The listing builds one solid part. Answer for the finished solid, in the listing's coordinates (mm). Coordinates: 2 decimals unless noted, no trailing zeros. Order: outer loops, then holes, each group sorted by start corner. A loop starts at its lowest first (then second) coordinate and runs counter-clockwise, first axis right, second up. Notation, with made-up numbers: (-36, 81.25) - (22, 81.25) arc R13 ccw to (22, 103.25) - close; hole circle Ø2 at (48, 0). An arc over 180 degrees is marked (long way). One line per item, written item: value. Start each with the question number.
```python
from build123d import *

# Parameters (mm, degrees)
F0_W     = 152.4
F0_H     = 14.740049
F0_H_2   = 8.316415
F0_H_3   = 8.693536
F1_DEPTH = 3.175
F2_DEPTH = 55.118
F3_W     = 38.1
F3_H     = 9.525
F4_DEPTH = 25.4


with BuildPart() as f1:
    # F0 (on Top) → F1 (new body)
    with BuildSketch(Plane.XY):
        with Locations((77.322651, 15.686439)):
            Rectangle(F0_W, F0_H)
        with Locations((77.322651, 4.158207)):
            Rectangle(F0_W, F0_H_2)
        with Locations((77.322651, -4.346768)):
            Rectangle(F0_W, F0_H_3)
    extrude(amount=F1_DEPTH)

    # F0 (on Top) → F2 (cut)
    with BuildSketch(Plane.XY):
        with Locations((77.322651, 4.158207)):
            Rectangle(F0_W, F0_H_2)
    extrude(amount=-F2_DEPTH, mode=Mode.SUBTRACT)

    # F3 (on face) → F4 (cut)
    with BuildSketch(Plane.XY.offset(3.175)):
        with Locations((38.663851, 7.181464)):
            Rectangle(F3_W, F3_H)
    extrude(amount=-F4_DEPTH, mode=Mode.SUBTRACT)


solid = f1.part
```
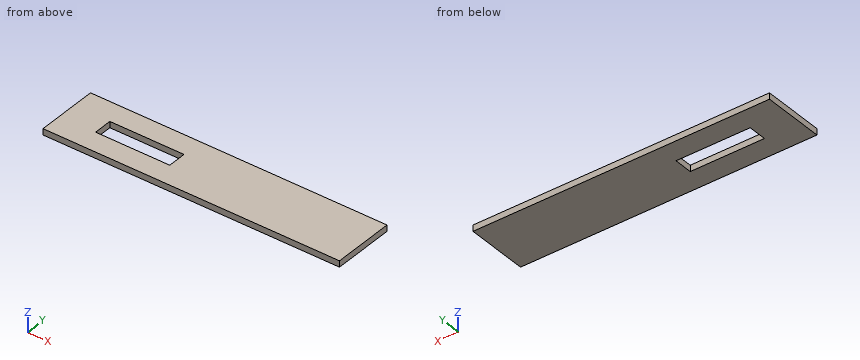
(1) Consider probe 1 along Y at (x, z) = (50, 0.6); probe 2 along X at (y, z) = (11, 2.55). Determine where each line is inside the solid, lowest interval first.
(2) The part is cut by section A-A on y = 8.5. Determine the outline of the cut face in (x, z) (3 decimals).
(3) The part is cut by section B-B on x = 25. Determine the outline of the cut face in (y, z) (3 decimals).
(4) The part is cut by section C-C on z = 0.9. Determine the outline of the cut face in (x, y).
Completed:
1. probe 1: y = -8.69 to 2.42, 11.94 to 23.06
1. probe 2: x = 1.12 to 19.61, 57.71 to 153.52
2. outline: (1.123, 0) - (19.614, 0) - (19.614, 3.175) - (1.123, 3.175) - close; (57.714, 0) - (153.523, 0) - (153.523, 3.175) - (57.714, 3.175) - close
3. outline: (-8.694, 0) - (2.419, 0) - (2.419, 3.175) - (-8.694, 3.175) - close; (11.944, 0) - (23.056, 0) - (23.056, 3.175) - (11.944, 3.175) - close
4. outline: (1.12, -8.69) - (153.52, -8.69) - (153.52, 23.06) - (1.12, 23.06) - close; hole (19.61, 2.42) - (57.71, 2.42) - (57.71, 11.94) - (19.61, 11.94) - close
